from build123d import *

# Parameters (mm, degrees)
CUT_EXTRUDE1_REACH = 8.695
CIRPATTERN1_COUNT  = 4
DRAFT1_ANGLE       = 5
CHAMFER1_SIZE      = 0.133096
CHAMFER1_SIZE2     = 0.121906137


with BuildPart() as part:
    # Sketch2 → Revolve1 (revolve)
    with BuildSketch(Plane.XY, mode=Mode.PRIVATE) as revolve1_sk:
        Polygon((-2.38125, 0), (2.38125, 0), (2.38125, 1.7526), (-0.88265, 1.7526), (-0.88265, 2.024686895), (-2.38125, 3.3274), align=None)
    revolve(revolve1_sk.sketch.rotate(Axis((-2.38125, 0, 0), (1, 0, 0)), 180), axis=Axis((-2.38125, 0, 0), (1, 0, 0)))

    # Cut-Extrude1: up to this cone (the profile starts inside it)
    cut_extrude1_end = Plane(origin=(-2.38125, 0, 0), z_dir=(-1, 0, 0)).offset(-2.137134931) * Cone(1e-06, 11.465822401, 13.189918853, align=(Align.CENTER, Align.CENTER, Align.MIN), mode=Mode.PRIVATE)
    # Sketch3 → Cut-Extrude1 (cut, up to the surface)
    with BuildSketch(Plane.ZY.offset(2.38125), mode=Mode.PRIVATE) as cut_extrude1_sk1:
        with BuildLine():
            Line((0, 0), (2.218266667, 0))
            ThreePointArc((2.218266667, 0), (2.207033704, 0.22295568), (2.173448579, 0.443653333))
            Line((2.173448579, 0.443653333), (1.308550956, 0.443653333))
            Line((1.308550956, 0.443653333), (0.696975982, 0.696975982))
            Line((0.696975982, 0.696975982), (0.443653333, 1.308550956))
            Line((0.443653333, 1.308550956), (0.443653333, 2.173448579))
            ThreePointArc((0.443653333, 2.173448579), (0.22295568, 2.207033704), (0, 2.218266667))
            Line((0, 2.218266667), (0, 0))
        make_face()
    cut_extrude1_tool1 = extrude(cut_extrude1_sk1.sketch, amount=-CUT_EXTRUDE1_REACH, mode=Mode.PRIVATE) & cut_extrude1_end
    cut_extrude1 = cut_extrude1_tool1.solids().sort_by_distance((-2.38125, 1.109133, 0.031371))[0]
    add(cut_extrude1, mode=Mode.SUBTRACT)

    # CirPattern1: Cut-Extrude1 ×4 about axis
    cirpattern1_axis = Axis((0, 0, 0), (1, 0, 0))
    for i in range(1, CIRPATTERN1_COUNT):
        add(cut_extrude1.rotate(cirpattern1_axis, i * 360 / CIRPATTERN1_COUNT), mode=Mode.SUBTRACT)

    # Draft1
    draft1_faces = [part.faces().sort_by_distance(p)[0] for p in [
        (-2.19829002, 0.443653333, -1.474018434),
        (-1.970823894, 0.582482874, -0.973386795),
        (-1.970823894, 0.973386795, -0.582482874),
        (-2.19829002, 1.474018434, -0.443653333),
        (-2.19829002, 1.474018434, 0.443653333),
        (-1.970823894, 0.973386795, 0.582482874),
        (-1.970823894, 0.582482874, 0.973386795),
        (-2.19829002, 0.443653333, 1.474018434),
        (-2.19829002, -0.443653333, 1.474018434),
        (-1.970823894, -0.582482874, 0.973386795),
        (-1.970823894, -0.973386795, 0.582482874),
        (-2.19829002, -1.474018434, 0.443653333),
        (-2.19829002, -1.474018434, -0.443653333),
        (-1.970823894, -0.973386795, -0.582482874),
        (-1.970823894, -0.582482874, -0.973386795),
        (-2.19829002, -0.443653333, -1.474018434),
    ]]
    draft(draft1_faces, Plane(origin=(-2.38125, 0, 0), x_dir=(0, -1, 0), z_dir=(-1, 0, 0)), DRAFT1_ANGLE)

    # Chamfer1
    chamfer1_edges = [part.edges().sort_by_distance(p)[0] for p in [
        (-2.38125, 3.3274, 0),
    ]]
    chamfer1_side = [part.faces().sort_by_distance(p)[0] for p in [
        (-1.63195, 2.676043447, 0),
    ]]
    chamfer(chamfer1_edges, length=CHAMFER1_SIZE, length2=CHAMFER1_SIZE2, reference=chamfer1_side[0])


solid = part.part
Read the model definition and answer for the solid it produces. Units are mm, in the model's axes. Give positions to 0.01 mm unless a question says otherwise; leave off trailing zeros. Write each loop counter-clockwise with the first axis right and the second up, starting at its lowest first coordinate (ties: lowest second). Pieces come first, ordered by that corner, then holes. Notation, with made-up numbers: (71, -16.75) - (109, -16.75) arc R15 cw to (109, 9.25) - close; hole circle Ø6 at (57, -16.75). An arc over 180 degrees is marked (long way). Use CSV: the item, a comma, the result in double quotes. Start each with the question number.
Item 1: The part is cut by section B-B, the plane x = 2.05. Give the vertices of the cut face in (y, z), and give its area (3 significant figures).
Item 2: Flat-ended cylindrical pins translate along their axes: P1, Ø1.5, axis at x = -1, y = -0.5, coming from the +Z side; P2, Ø1, axis at x = -1, z = 1.5, coming from the +Y side. Find the tip coordinate at first contact, or state that the pin passes through.
Item 3: Consider line 1 (Y direction, x = -1.3, z = -0.5); line 2 (X direction, y = 0, z = -2); line 3 (Z direction, x = -1.9, y = 0.5). Determine where each line is inside the solid, lowest interval first.
Item 4: The part is cut by section C-C, the plane x = -0.65. Give the vertices of the cut face in (y, z), and give its area (3 significant figures).
Item 5: The part is cut by section A-A, the plane x = -1.65. Give the vertices of the cut face in (y, z), and give its area (3 significant figures).
Item 6: The mould has two halves that part along Y. Classify faces 1 (the conical face through (-0.853, -0.023, 0.529)), 2 (the cylindrical face through (0.73, -1.67, -0.53)), 3 (the flat face through (2.381, 0, 0)): pulls with the +Y half, pulls with the -Y half, needs draft (parallel to the pull), parting line crosses it, or undercut.
Taken from the geometry:
1,outline,"circle Ø3.51 at (0, 0)"
1,area,"9.65 mm2"
2,P1,"z = 2.74"
2,P2,"y = 2.17"
3,line 1,"-2.33 to -0.77, 0.77 to 2.33"
3,line 2,"-2.38 to -0.88"
3,line 3,"-2.87 to -1.06, 1.06 to 2.87"
4,outline,"circle Ø3.51 at (0, 0); hole circle Ø0.71 at (0, 0)"
4,area,"9.26 mm2"
5,outline,"circle Ø5.38 at (0, 0); hole (-1.14, -0.44) - (-0.65, -0.65) - (-0.44, -1.14) arc R1.22 ccw to (0.44, -1.14) - (0.65, -0.65) - (1.14, -0.44) arc R1.22 ccw to (1.14, 0.44) - (0.65, 0.65) - (0.44, 1.14) arc R1.22 ccw to (-0.44, 1.14) - (-0.65, 0.65) - (-1.14, 0.44) arc R1.22 ccw to start"
5,area,"18.7 mm2"
6,face 1,"undercut"
6,face 2,"parting line crosses it"
6,face 3,"needs draft"
